Can you work these out from the model? Positions are in its coordinate system, mm. A direction names the side the tool comes from. Round coordinates to 2 decimals unless told otherwise and drop trailing zeros. Loops run counter-clockwise (first coordinate to the right, second up) from the corner with the lowest first, then second, coordinate; pieces in that order, holes last. Notation, with made-up numbers: (26, 61.5) -> (61, 61.5) arc R24 cw to (61, 89.5) -> close; hole circle Ø9 at (66.25, 25.25). An arc over 180 degrees is marked (long way). Write item = value, one per line.
from build123d import *

# Parameters (mm, degrees)
F2_R      = 76.2
F5_DEPTH  = 609.6
F4_R      = 76.2
F6_DEPTH  = 304.8
F7_T      = -6.35
F7_2_T    = -6.35
F9_R      = 95.25
F9_R_2    = 76.2
F10_DEPTH = 12.7
F12_R     = 95.25
F12_R_2   = 76.2
F13_DEPTH = 12.7
F14_R     = 95.25
F14_R_2   = 76.2
F15_DEPTH = 12.7


with BuildPart() as f5:
    # F2 (on plane+point) → F5 (new body)
    with BuildSketch(Plane.XZ.offset(294.1361665726)):
        Circle(F2_R)
    extrude(amount=-F5_DEPTH)

    # F7
    f7_openings = [f5.faces().sort_by_distance(p)[0] for p in [
        (0, 315.463833, 0),
        (0, -294.136167, 0),
    ]]
    offset(amount=F7_T, openings=f7_openings)

    # F9 (on line) → F10 (join)
    with BuildSketch(Plane(origin=(0, -294.1361665726, 0), x_dir=(-1, 0, 0), z_dir=(0, 1, 0))):
        Circle(F9_R)
        Circle(F9_R_2, mode=Mode.SUBTRACT)
    extrude(amount=F10_DEPTH)

    # F12 (on line) → F13 (join)
    with BuildSketch(Plane(origin=(0, 315.4638334274, 0), x_dir=(-1, 0, 0), z_dir=(0, 1, 0))):
        Circle(F12_R)
        Circle(F12_R_2, mode=Mode.SUBTRACT)
    extrude(amount=-F13_DEPTH)



with BuildPart() as f6:
    # F4 (on plane+point) → F6 (new body)
    with BuildSketch(Plane.XY.offset(304.8)):
        Circle(F4_R)
    extrude(amount=-F6_DEPTH)

    # F7#2
    f7_2_openings = [f6.faces().sort_by_distance(p)[0] for p in [
        (0, 0, 304.8),
    ]]
    offset(amount=F7_2_T, openings=f7_2_openings)


with BuildPart() as f5_1:
    add(f5.part)

    add(f6.part)  # F15 merges F6
    # F14 (on plane+point) → F15 (join)
    with BuildSketch(Plane.XY.offset(304.8)):
        Circle(F14_R)
        Circle(F14_R_2, mode=Mode.SUBTRACT)
    extrude(amount=-F15_DEPTH)


solid = f5_1.part
1. Suppose I cut it at D-D, the plane z = -9. List the corners of the cut face in (x, y) for me.
Entries:
outline = (-94.82, -294.14) -> (-69.27, -294.14) -> (-69.27, 315.46) -> (-94.82, 315.46) -> (-94.82, 302.76) -> (-75.67, 302.76) -> (-75.67, -281.44) -> (-94.82, -281.44) -> close; (69.27, -294.14) -> (94.82, -294.14) -> (94.82, -281.44) -> (75.67, -281.44) -> (75.67, 302.76) -> (94.82, 302.76) -> (94.82, 315.46) -> (69.27, 315.46) -> close
2. I'm going to push flat-ended pins straight in: pin 1 (5 mm diameter, centred on x = 55.5, z = 18, fed in from -Y); pin 2 (4 mm diameter, centred on y = -0.5, z = -54.5, fed in from -X); pin 3 (4 mm diameter, centred on x = -66, y = 96, fed in from +Z). Where does each tip first touch, or does it pass through?
Entries:
pin_1 = -54.75
pin_2 = -55.23
pin_3 = 41.36
3. I need wall thicknesses on line 1 (Z direction, x = 2, y = -81); line 2 (Z direction, x = 0, y = -15.5); line 3 (Y direction, x = -80.5, z = -31.5). Which ranges of each line are inside material? Lowest first, please. Write a range as [from, to].
Entries:
line_1 = [-76.17, -69.82], [69.82, 76.17], [292.1, 304.8]
line_2 = [-76.2, -69.85], [0, 6.35], [69.85, 76.2]
line_3 = [-294.14, -281.44], [302.76, 315.46]
4. Suppose I cut it at A-A, the plane y = 0. List the corners of the cut face in (x, z) for me, and give its area (3 significant figures).
Entries:
outline = (-95.25, 292.1) -> (-76.2, 292.1) -> (-76.2, 0) arc R76.2 ccw to (76.2, 0) -> (76.2, 292.1) -> (95.25, 292.1) -> (95.25, 304.8) -> (69.85, 304.8) -> (69.85, 30.45) arc R76.2 ccw to (-69.85, 30.45) -> (-69.85, 304.8) -> (-95.25, 304.8) -> close; hole (-69.85, 0) arc R69.85 ccw to (69.85, 0) -> close; hole (-69.56, 6.35) -> (69.56, 6.35) arc R69.85 ccw to start
area = 7,890 mm²
5. Suppose I cut it at B-B, the plane x = 0. Count the separate pieces of the cut face and the enclosed holes in it, and give its area (3 significant figures).
Entries:
separate_pieces = 2
enclosed_holes = 1
area = 13,900 mm²
6. We'd pull the mould along Y, two halves only. Please class faces 4 (the flat face through (29, 315.464, 64)), 5 (the cylindrical face through (75.587, -287.875, -57.958)), 6 (the cylindrical face through (1.24, -0.98, 76.19)): released by +Y, released by -Y, zero draft, split by the parting line, or undercut.
Entries:
face_4 = released by +Y
face_5 = zero draft
face_6 = undercut
7. Suppose I cut it at C-C, the plane z = 136. List the corners of the cut face in (x, y) for me, and give its area (3 significant figures).
Entries:
outline = circle Ø152.4 at (0, 0); hole circle Ø139.7 at (0, 0)
area = 2,910 mm²
8. For faces 1 (the cylindrical face through (-60.47, -46.367, 180.55)), 2 (the cylindrical face through (64.524, -26.753, 169.547)), 3 (the flat face through (29, -294.136, 64)), which set-ups out of +Z, -Z, +X, -X, +Y, -Y let a thin tool reach every point of the face, with its end or its side?
Entries:
face_1 = none
face_2 = +Z
face_3 = +Z, -Z, +X, -X, -Y
